Geometry: see drawing. Coordinates: mm, zero at the bounding-box minimum. A direction names the side the tool comes from. Give positions to 0.01 mm unless a question says otherwise; leave off trailing zeros. Order: outer loops, then holes, each group sorted by start corner. A loop starts at its lowest first (then second) coordinate and runs counter-clockwise, first axis right, second up. Notation, with made-up numbers: M 75,11 L 109,11 A7 ccw 109,15 Z; hole C -25,-4.75 d1. An arc over 180 degrees is marked long. Use a Markdown table: item, result.
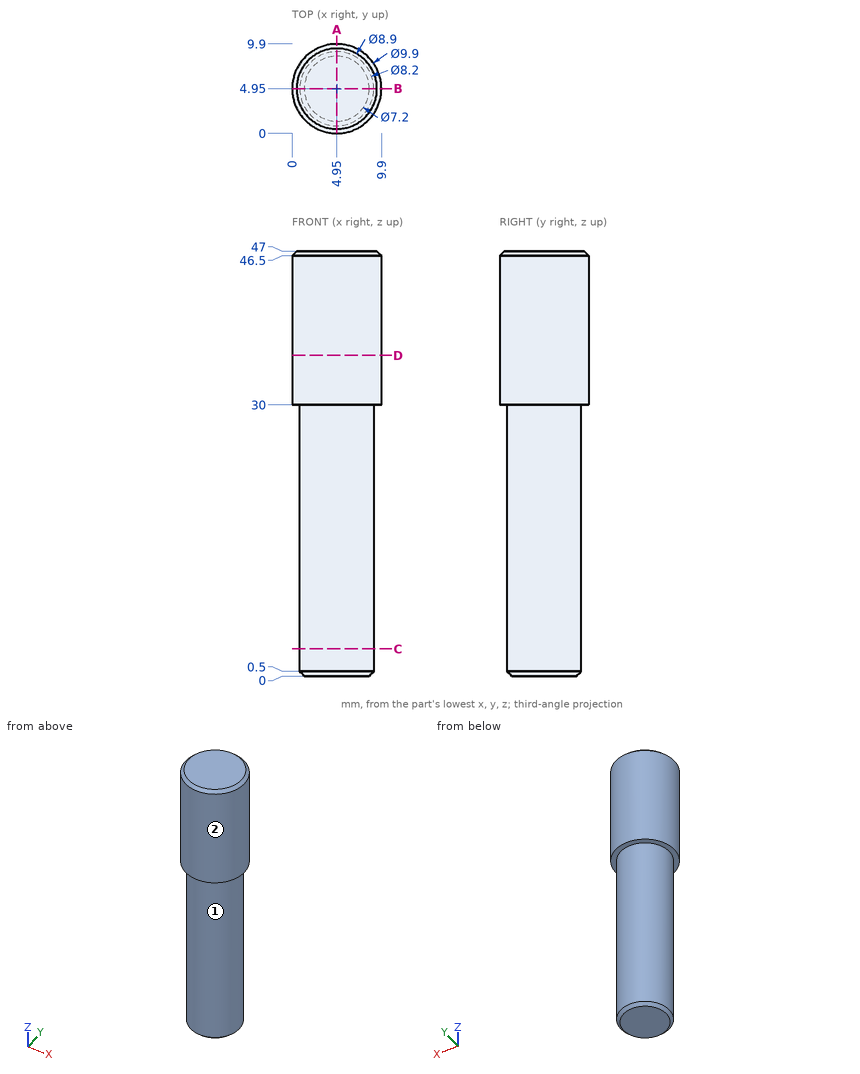
1) First-contact query: pin 1 Ø3 at (x, z) = (9, 33.5) entering from +Y; pin 2 Ø4 at (y, z) = (7.5, 30.5) entering from -X. Flat tips, straight axial feed; report the tip coordinate or a pass-through.
Response values:
| item | result |
|---|---|
| pin 1 | stops at y = 9.19 |
| pin 2 | stops at x = 0.03 |
2) Cut plane A-A on x = 4.95. Return loops of the section in (y, z), and give its area (3 significant figures).
Response values:
| item | result |
|---|---|
| outline | M 0,30 L 0.85,30 L 0.85,0.5 L 1.35,0 L 8.55,0 L 9.05,0.5 L 9.05,30 L 9.9,30 L 9.9,46.5 L 9.4,47 L 0.5,47 L 0,46.5 Z |
| area | 414 mm² |
3) Material intervals for line 1 (X direction, y = 4.75, z = 21); line 2 (Y direction, x = 3, z = 2.5), sorted ascending. Write a range as from..to.
Response values:
| item | result |
|---|---|
| line 1 | x = 0.85..9.05 |
| line 2 | y = 1.34..8.56 |
4) Reachability of the marked faces 1 and 2 from +Z, -Z, +X, -X, +Y, -Y: full face, straight path, thin tool, end or side. Return the list, or none.
Response values:
| item | result |
|---|---|
| face 1 | -Z |
| face 2 | +Z, -Z |
5) Cut plane D-D on z = 35.5. Return loops of the section in (x, y).
Response values:
| item | result |
|---|---|
| outline | C 4.95,4.95 d9.9 |
6) Cut plane C-C on z = 3. Return loops of the section in (x, y).
Response values:
| item | result |
|---|---|
| outline | C 4.95,4.95 d8.2 |
